```python
from build123d import *

# Parameters (mm, degrees)
BOX001_W               = 10
BOX001_H               = 10
BOX001_DEPTH           = 10
BOX001_PLACEMENT_ANGLE = 315
BOX004_W               = 10
BOX004_H               = 10
BOX004_DEPTH           = 0.5
BOX005_W               = 10
BOX005_H               = 10
BOX005_DEPTH           = 0.5
BOX006_W               = 10
BOX006_H               = 10
BOX006_DEPTH           = 0.5
BOX003_W               = 1.7
BOX003_H               = 10
BOX003_DEPTH           = 4
BOX002_W               = 3
BOX002_H               = 3
BOX002_DEPTH           = 4
BOX_W                  = 10
BOX_H                  = 10
BOX_DEPTH              = 10
CYLINDER_R             = 2
CYLINDER_DEPTH         = 10


with BuildPart() as angle_cutter:
    # Box001 → Box001 (new body)
    with BuildSketch(Plane.XY):
        with Locations((5, 5)):
            Rectangle(BOX001_W, BOX001_H)
    extrude(amount=BOX001_DEPTH)


with BuildPart() as angle_cutter_1:
    # Box001 placement: moved
    add(angle_cutter.part.moved(Location((-5, -7.5, -5.5))).rotate(Axis((-5, -7.5, -5.5), (1, 0, 0)), BOX001_PLACEMENT_ANGLE))


with BuildPart() as cube003:
    # Box004 → Box004 (new body)
    with BuildSketch(Plane(origin=(-1, -5, 4), x_dir=(1, 0, 0), z_dir=(0, 0, 1))):
        with Locations((5, 5)):
            Rectangle(BOX004_W, BOX004_H)
    extrude(amount=BOX004_DEPTH)


with BuildPart() as cube004:
    # Box005 → Box005 (new body)
    with BuildSketch(Plane(origin=(-9, -2, 3), x_dir=(1, 0, 0), z_dir=(0, 0, 1))):
        with Locations((5, 5)):
            Rectangle(BOX005_W, BOX005_H)
    extrude(amount=BOX005_DEPTH)


with BuildPart() as fusion001:
    # Box006 → Box006 (new body)
    with BuildSketch(Plane(origin=(-5, -11, 2), x_dir=(1, 0, 0), z_dir=(0, 0, 1))):
        with Locations((5, 5)):
            Rectangle(BOX006_W, BOX006_H)
    extrude(amount=BOX006_DEPTH)

    # Fusion001: union Cube003, Cube004
    add(cube003.part)
    add(cube004.part)


with BuildPart() as cube002:
    # Box003 → Box003 (new body)
    with BuildSketch(Plane(origin=(-0.85, -4, 4), x_dir=(1, 0, 0), z_dir=(0, 0, 1))):
        with Locations((0.85, 5)):
            Rectangle(BOX003_W, BOX003_H)
    extrude(amount=BOX003_DEPTH)


with BuildPart() as fusion:
    # Box002 → Box002 (new body)
    with BuildSketch(Plane(origin=(-1.5, -4, 4), x_dir=(1, 0, 0), z_dir=(0, 0, 1))):
        with Locations((1.5, 1.5)):
            Rectangle(BOX002_W, BOX002_H)
    extrude(amount=BOX002_DEPTH)

    # Fusion: union Cube002
    add(cube002.part)


with BuildPart() as fusion_1:
    # Fusion placement: moved
    add(fusion.part.moved(Location((0, 0, 1))))


with BuildPart() as cube:
    # Box → Box (new body)
    with BuildSketch(Plane(origin=(-5, -0.5, 0), x_dir=(1, 0, 0), z_dir=(0, 0, 1))):
        with Locations((5, 5)):
            Rectangle(BOX_W, BOX_H)
    extrude(amount=BOX_DEPTH)


with BuildPart() as cut003:
    # Cylinder → Cylinder (new body)
    with BuildSketch(Plane.XY):
        Circle(CYLINDER_R)
    extrude(amount=CYLINDER_DEPTH)

    # Cut: cut Cube
    add(cube.part, mode=Mode.SUBTRACT)

    # Cut001: cut Fusion
    add(fusion_1.part, mode=Mode.SUBTRACT)

    # Cut002: cut Fusion001
    add(fusion001.part, mode=Mode.SUBTRACT)

    # Cut003: cut Angle Cutter
    add(angle_cutter_1.part, mode=Mode.SUBTRACT)


solid = cut003.part
```
Verification items for the finished model (mm, model axes). A direction names the side the tool comes from. Coordinates: 2 decimals unless noted, no trailing zeros. Write each loop counter-clockwise with the first axis right and the second up, starting at its lowest first coordinate (ties: lowest second). Pieces come first, ordered by that corner, then holes. Notation, with made-up numbers: M -36,34.25 L -30,34.25 A21 ccw -30,57.25 Z; hole C 27,-29 d6. An arc over 180 degrees is marked long. Answer as a JSON object with one key per item and string values. Group by question number.
(1) Material ranges on line 1 (Z direction, x = -0.7, y = -1.7); line 2 (Z direction, x = -0.5, y = -1.45); line 3 (Y direction, x = -1.1, z = 8), recorded low to high.
(2) Release check for a two-part mould opening along Z. For faces 1 (the face through (0, -1, 1)), 2 (the face through (0, -0.5, 4.7)), 3 (the face through (0, -1, 4)) record: +Z half, -Z half, draft (parallel to the pull), parting line (faces both ways), or undercut.
(3) Cross-section at A-A, the plane y = -1.2. Record the cut outline in (x, z).
(4) Cross-section at D-D, the plane x = -0.3. Record the cut outline in (y, z).
(5) Cross-section at B-B, the plane z = 5.75. Record the cut outline in (x, y).
(6) Tool access check on faces 4 (the face through (0, -1, 5)), 5 (the face through (0, -1, 3)), 6 (the face through (0, -1.4, 2)), 7 (the face through (0, -1, 4.5)), 8 (the face through (0, -1, 10)). Record the directions out of +Z, -Z, +X, -X, +Y, -Y that give a thin tool (end or side, any length) a straight path to the whole face; none if there is none.
(7) Gauge pin test, flat ends, axial feed: pin 1 (0.6 mm diameter, centred on y = -1.5, z = 4, fed in from +X); pin 2 (0.8 mm diameter, centred on x = -0.5, y = -1.5, fed in from -Z). Record the tip position at first contact, or that the pin passes through.
(8) Cross-section at C-C, the plane x = -1.6. Record the cut outline in (y, z).
Reply:
{
 "1": {"line 1": "0.3 to 2, 2.5 to 3, 3.5 to 4, 4.5 to 5, 9 to 10", "line 2": "0.55 to 2, 2.5 to 3, 3.5 to 4, 4.5 to 5, 9 to 10", "line 3": "-1 to -0.5"},
 "2": {"face 1": "-Z half", "face 2": "draft", "face 3": "undercut"},
 "3": {"outline": "M -1.6,0.8 L 1.6,0.8 L 1.6,2 L -1.6,2 Z; M -1.6,2.5 L 1.6,2.5 L 1.6,4 L -1,4 L -1,4.5 L 1.6,4.5 L 1.6,10 L -1.6,10 L -1.6,3.5 L 1,3.5 L 1,3 L -1.6,3 Z; hole M -1.5,5 L 1.5,5 L 1.5,9 L -1.5,9 Z"},
 "4": {"outline": "M -1.98,0.02 L -0.5,1.5 L -0.5,3 L -1.98,3 L -1.98,2.5 L -1,2.5 L -1,2 L -1.98,2 Z; M -1.98,3.5 L -0.5,3.5 L -0.5,4 L -1.98,4 Z; M -1.98,4.5 L -0.5,4.5 L -0.5,5 L -1.98,5 Z; M -1.98,9 L -0.5,9 L -0.5,10 L -1.98,10 Z"},
 "5": {"outline": "M -1.94,-0.5 A2 ccw -1.5,-1.32 L -1.5,-1 L -0.85,-1 L -0.85,-0.5 Z; M 0.85,-1 L 1.5,-1 L 1.5,-1.32 A2 ccw 1.94,-0.5 L 0.85,-0.5 Z"},
 "6": {"face 4": "-Y", "face 5": "-X, +Y, -Y", "face 6": "+X, -X, -Y", "face 7": "+X, +Y, -Y", "face 8": "+Z, +X, -X, +Y, -Y"},
 "7": {"pin 1": "x = 1.6", "pin 2": "z = 0.1"},
 "8": {"outline": "M -1.2,0.8 L -0.5,1.5 L -0.5,3 L -1.2,3 L -1.2,2.5 L -1,2.5 L -1,2 L -1.2,2 Z; M -1.2,3.5 L -0.5,3.5 L -0.5,10 L -1.2,10 Z"}
}
